Geometry check sheet. Reference: the model listing, model coordinates, mm. Face numbers are marked on the shaded views. A direction names the side the tool comes from. Round coordinates to 2 decimals unless told otherwise and drop trailing zeros. Loops run counter-clockwise (first coordinate to the right, second up) from the corner with the lowest first, then second, coordinate; pieces in that order, holes last. Notation, with made-up numbers: (36, 66.5) - (65, 66.5) arc R3 cw to (65, 71.5) - close; hole circle Ø8 at (16, 26.25). An arc over 180 degrees is marked (long way). Write item = value, one per line.
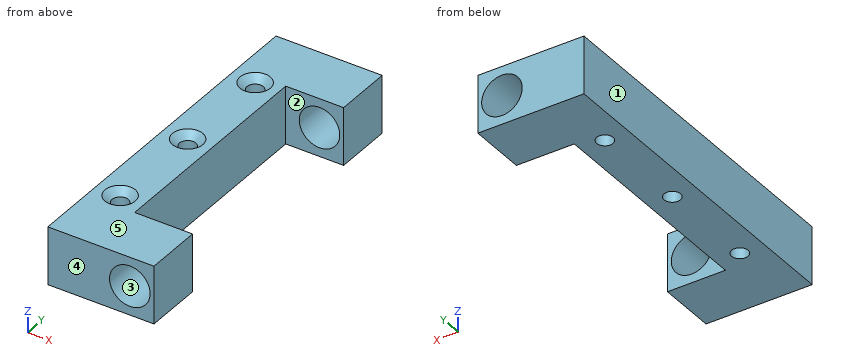
```python
from build123d import *

# Parameters (mm, degrees)
AUFSATZ_LINEAR_AUSTRAGEN1_DEPTH                      = 12
FORMSENKUNG_F_R_M3_LINSENSENKSCHRAUBE_MI_D           = 3.4
FORMSENKUNG_F_R_M3_LINSENSENKSCHRAUBE_MI_CSINK_D     = 6.3
FORMSENKUNG_F_R_M3_LINSENSENKSCHRAUBE_MI_CSINK_ANGLE = 90
F_8_4_8_4_DURCHMESSER_BOHRUNG3_D                     = 8.4


with BuildPart() as part:
    # Skizze1 → Aufsatz-Linear austragen1 (new body)
    with BuildSketch(Plane.XY):
        Polygon((0, 0), (0, 71), (22, 71), (22, 59), (10, 59), (10, 12), (22, 12), (22, 0), align=None)
    extrude(amount=AUFSATZ_LINEAR_AUSTRAGEN1_DEPTH)

    # Formsenkung für M3 Linsensenkschraube mit Schlitz2 (through all)
    with Locations(Plane.XY.offset(12)):
        with Locations((5, 57), (5, 36), (5, 15)):
            CounterSinkHole(FORMSENKUNG_F_R_M3_LINSENSENKSCHRAUBE_MI_D / 2, FORMSENKUNG_F_R_M3_LINSENSENKSCHRAUBE_MI_CSINK_D / 2, counter_sink_angle=FORMSENKUNG_F_R_M3_LINSENSENKSCHRAUBE_MI_CSINK_ANGLE)

    # Ø8.4 (8.4) Durchmesser Bohrung3 (through all)
    with Locations(Plane(origin=(0, 71, 0), x_dir=(1, 0, 0), z_dir=(0, 1, 0))):
        with Locations((17, -6)):
            Hole(F_8_4_8_4_DURCHMESSER_BOHRUNG3_D / 2)


solid = part.part
```
(1) Section check C-C (y = 57). Enter the section's corners in (x, z).
Answers follow:
outline = (0, 0) - (3.3, 0) - (3.3, 10.55) - (1.85, 12) - (0, 12) - close; (6.7, 0) - (10, 0) - (10, 12) - (8.15, 12) - (6.7, 10.55) - close
(2) Section check D-D (z = 3.5). Enter the section's corners in (x, y), then the cut area to 3 significant figures.
Answers follow:
outline = (0, 0) - (13.63, 0) - (13.63, 12) - (10, 12) - (10, 59) - (13.63, 59) - (13.63, 71) - (0, 71) - close; (20.37, 0) - (22, 0) - (22, 12) - (20.37, 12) - close; (20.37, 59) - (22, 59) - (22, 71) - (20.37, 71) - close; hole circle Ø3.4 at (5, 15); hole circle Ø3.4 at (5, 36); hole circle Ø3.4 at (5, 57)
area = 809 mm²
(3) Gauge pin test, flat ends, axial feed: pin 1 (6 mm diameter, centred on y = 47, z = 3, fed in from +X); pin 2 (1.5 mm diameter, centred on x = 18.5, z = 6.5, fed in from -Y); pin 3 (4.5 mm diameter, centred on x = 5, y = 36, fed in from +Z). Record the tip position at first contact, or that the pin passes through.
Answers follow:
pin_1 = 10
pin_2 = through
pin_3 = 11.1
(4) Set-up check for the marked faces 1 and 2: record each of +Z, -Z, +X, -X, +Y, -Y from which the full face is reachable in a straight line by a thin tool's end or side.
Answers follow:
face_1 = +Z, -Z, -X, +Y, -Y
face_2 = +Z, -Z, +X
(5) Section check A-A (x = 17). Enter the section's corners in (y, z), then the cut area to 3 significant figures.
Answers follow:
outline = (0, 0) - (12, 0) - (12, 1.8) - (0, 1.8) - close; (0, 10.2) - (12, 10.2) - (12, 12) - (0, 12) - close; (59, 0) - (71, 0) - (71, 1.8) - (59, 1.8) - close; (59, 10.2) - (71, 10.2) - (71, 12) - (59, 12) - close
area = 86.4 mm²
(6) Scan lines: L1, parallel to Z at x = 17, y = 67.75; L2, parallel to Y at x = 13.25, z = 1; L3, parallel to X at y = 15, z = 5.5. Record each from-to range of solid material in increasing order. Write a range as [from, to].
Answers follow:
L1 = [0, 1.8], [10.2, 12]
L2 = [0, 12], [59, 71]
L3 = [0, 3.3], [6.7, 10]
(7) Section check B-B (z = 7.25). Enter the section's corners in (x, y), then the cut area to 3 significant figures.
Answers follow:
outline = (0, 0) - (12.99, 0) - (12.99, 12) - (10, 12) - (10, 59) - (12.99, 59) - (12.99, 71) - (0, 71) - close; (21.01, 0) - (22, 0) - (22, 12) - (21.01, 12) - close; (21.01, 59) - (22, 59) - (22, 71) - (21.01, 71) - close; hole circle Ø3.4 at (5, 15); hole circle Ø3.4 at (5, 36); hole circle Ø3.4 at (5, 57)
area = 778 mm²
(8) Mould release check, pull along Z, two halves, no side actions. Record for the marked faces 3, 4 and 5: pulls with the +Z half, pulls with the -Z half, needs draft (parallel to the pull), parting line crosses it, or undercut.
Answers follow:
face_3 = undercut
face_4 = needs draft
face_5 = pulls with the +Z half
